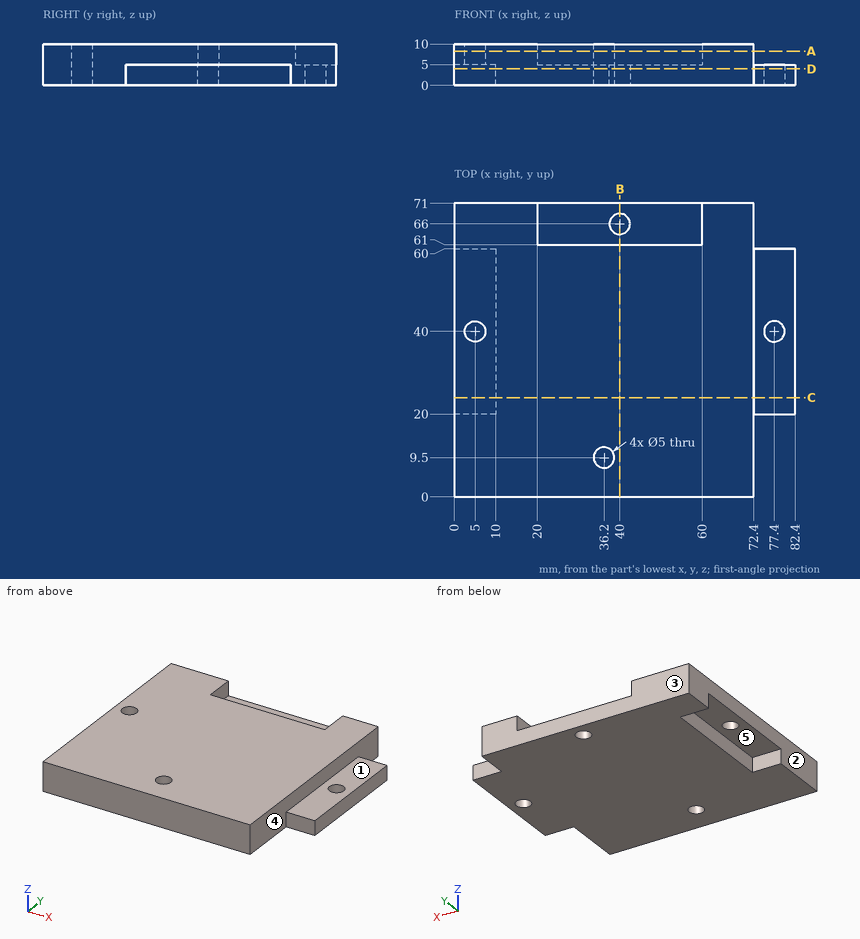
Source: three-view drawing plus pictorial views. Frame: mm from the lowest corner of the part. A direction names the side the tool comes from. Give positions to 0.01 mm unless a question says otherwise; leave off trailing zeros. Order: outer loops, then holes, each group sorted by start corner. A loop starts at its lowest first (then second) coordinate and runs counter-clockwise, first axis right, second up.
1. Pin query (flat end, axial travel): pin 1 (5.5 mm diameter, centred on x = 79.5, z = 3, fed in from -Y); pin 2 (3 mm diameter, centred on x = 75, y = 48, fed in from +Z); pin 3 (11 mm diameter, centred on x = 4, y = 34.5, fed in from -Z). Return the tip coordinate at first contact, or that it passes through.
Derived:
pin 1: stops at y = 20
pin 2: stops at z = 5
pin 3: stops at z = 5
2. Section A-A on z = 8.25. Return the cut outline in (x, y), and give its area (3 significant figures).
Derived:
outline: (0, 0) - (72.4, 0) - (72.4, 71) - (60, 71) - (60, 61) - (20, 61) - (20, 71) - (0, 71) - close; hole circle Ø5 at (5, 40); hole circle Ø5 at (36.2, 9.5)
area: 4,700 mm2
3. Material intervals for L1, parallel to X at y = 62, z = 7.5; L2, parallel to Y at x = 36.2, z = 7.5; L3, parallel to Y at x = 40, z = 3.4, sorted ascending.
Derived:
L1: x = 0 to 20, 60 to 72.4
L2: y = 0 to 7, 12 to 61
L3: y = 0 to 63.5, 68.5 to 71
4. Section C-C on y = 24. Return the cut outline in (x, z), and give its area (3 significant figures).
Derived:
outline: (0, 5) - (10, 5) - (10, 0) - (82.4, 0) - (82.4, 5) - (72.4, 5) - (72.4, 10) - (0, 10) - close
area: 724 mm2
5. Section B-B on x = 40. Return the cut outline in (y, z), and give its area (3 significant figures).
Derived:
outline: (0, 0) - (63.5, 0) - (63.5, 5) - (61, 5) - (61, 10) - (0, 10) - close; (68.5, 0) - (71, 0) - (71, 5) - (68.5, 5) - close
area: 635 mm2
6. Reachability of the marked faces 1 and 2 from +Z, -Z, +X, -X, +Y, -Y: full face, straight path, thin tool, end or side. Return the list, or none.
Derived:
face 1: +Z, +X, +Y, -Y
face 2: +Z, -Z, -X, +Y, -Y
7. Section D-D on z = 4. Return the cut outline in (x, y).
Derived:
outline: (0, 0) - (72.4, 0) - (72.4, 20) - (82.4, 20) - (82.4, 60) - (72.4, 60) - (72.4, 71) - (0, 71) - (0, 60) - (10, 60) - (10, 20) - (0, 20) - close; hole circle Ø5 at (36.2, 9.5); hole circle Ø5 at (40, 66); hole circle Ø5 at (77.4, 40)
8. Mould query, pull axis Y, two halves, no side actions, for the marked faces 3, 4 and 5. Classes: released by +Y, released by -Y, zero draft, split by the parting line, or undercut.
Derived:
face 3: released by +Y
face 4: zero draft
face 5: undercut
